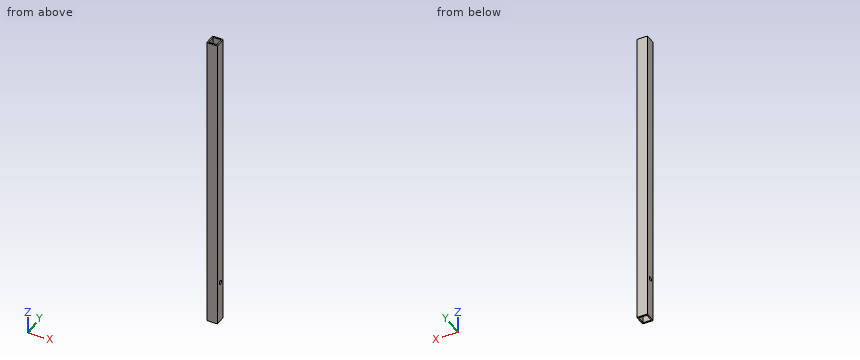
from build123d import *

# Parameters (mm, degrees)
SKETCH1_W           = 25.4
SKETCH1_H           = 25.4
SKETCH1_W_2         = 19.05
SKETCH1_H_2         = 19.05
BOSS_EXTRUDE1_DEPTH = 736.6
SKETCH3_R           = 4.7625
CUT_EXTRUDE1_DEPTH  = 127


with BuildPart() as part:
    # Sketch1 → Boss-Extrude1 (new body)
    with BuildSketch(Plane.XY):
        with Locations((3.05078858, 1.998217396)):
            Rectangle(SKETCH1_W, SKETCH1_H)
        with Locations((3.05078858, 1.998217396)):
            Rectangle(SKETCH1_W_2, SKETCH1_H_2, mode=Mode.SUBTRACT)
    extrude(amount=BOSS_EXTRUDE1_DEPTH)

    # Sketch3 → Cut-Extrude1 (cut)
    with BuildSketch(Plane.ZY.offset(9.64921142)):
        with Locations(Location((101.6, 1.998217396, 0), (0, 0, 270))):
            Circle(SKETCH3_R)
    extrude(amount=-CUT_EXTRUDE1_DEPTH, mode=Mode.SUBTRACT)


solid = part.part
The model under review builds one solid part; all positions refer to its coordinate system, in mm. Coordinates: 2 decimals unless noted, no trailing zeros. Write each loop counter-clockwise with the first axis right and the second up, starting at its lowest first coordinate (ties: lowest second). Pieces come first, ordered by that corner, then holes. Notation, with made-up numbers: (-24, 75.5) - (-11, 75.5) arc R20 cw to (-11, 81.5) - close; hole circle Ø4 at (66, -0.5). An arc over 180 degrees is marked (long way). Answer as a JSON object with one key per item and string values. Group by question number.
1. Clearance check with a flat-ended pin moving along its axis: pin 1 Ø2 at (x, y) = (-3.5, -2) entering from -Z. State where the tip first meets the part, or that it passes through.
2. Add section B-B (z = 179.5). Give the boundary of the cut face in (x, y).
3. To check wall thickness, follow probe 1 along X at (y, z) = (4.75, 270); probe 2 along Y at (x, z) = (-3.5, 682); probe 3 along Z at (x, y) = (-8.25, 4.5). State the ranges of each line that lie inside material, in increasing order.
4. Add section C-C (y = 1.5). Give the boundary of the cut face in (x, z).
5. Add section A-A (x = 0.75). Give the boundary of the cut face in (y, z).
Findings:
{
 "1": {"pin 1": "through"},
 "2": {"outline": "(-9.65, -10.7) - (15.75, -10.7) - (15.75, 14.7) - (-9.65, 14.7) - close; hole (-6.47, -7.53) - (12.58, -7.53) - (12.58, 11.52) - (-6.47, 11.52) - close"},
 "3": {"probe 1": "-9.65 to -6.47, 12.58 to 15.75", "probe 2": "-10.7 to -7.53, 11.52 to 14.7", "probe 3": "0 to 97.55, 105.65 to 736.6"},
 "4": {"outline": "(-9.65, 0) - (-6.47, 0) - (-6.47, 96.86) - (-9.65, 96.86) - close; (-9.65, 106.34) - (-6.47, 106.34) - (-6.47, 736.6) - (-9.65, 736.6) - close; (12.58, 0) - (15.75, 0) - (15.75, 96.86) - (12.58, 96.86) - close; (12.58, 106.34) - (15.75, 106.34) - (15.75, 736.6) - (12.58, 736.6) - close"},
 "5": {"outline": "(-10.7, 0) - (-7.53, 0) - (-7.53, 736.6) - (-10.7, 736.6) - close; (11.52, 0) - (14.7, 0) - (14.7, 736.6) - (11.52, 736.6) - close"}
}
